The drawing under review shows one solid part. Ordinate dimensions are in mm from its lowest x, y, z. Give positions to 0.01 mm unless a question says otherwise; leave off trailing zeros. Order: outer loops, then holes, each group sorted by start corner. A loop starts at its lowest first (then second) coordinate and runs counter-clockwise, first axis right, second up. Notation, with made-up numbers: (72, 30.5) -> (113, 30.5) arc R23 ccw to (113, 49.5) -> close; hole circle Ø3 at (-5, -9). An arc over 180 degrees is marked (long way). One line per item, written item: value.
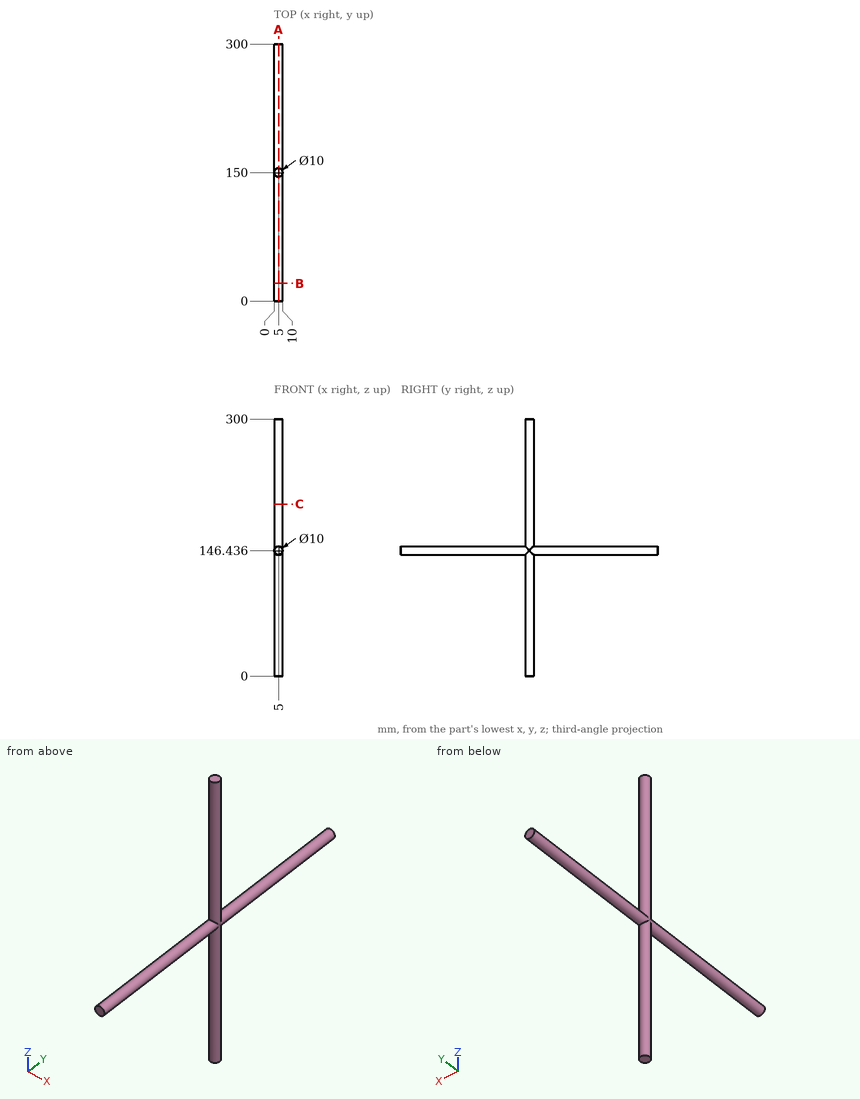
Item 1: Add section C-C on z = 200.5. Give the boundary of the cut face in (x, y).
Returned:
outline: circle Ø10 at (5, 150)
Item 2: Add section A-A on x = 5. Give the boundary of the cut face in (y, z) (1 decimal).
Returned:
outline: (0, 141.4) -> (145, 141.4) -> (145, 0) -> (155, 0) -> (155, 141.4) -> (300, 141.4) -> (300, 151.4) -> (155, 151.4) -> (155, 300) -> (145, 300) -> (145, 151.4) -> (0, 151.4) -> close
Item 3: To check wall thickness, follow line 1 along Z through (x, y) = (5.75, 99.5); line 2 along Y through (x, z) = (5, 135); line 3 along Y through (x, z) = (4.25, 154.5). State the ranges of each line that lie inside material, in increasing order. Write a range as from..to.
Returned:
line 1: 141.49..151.38
line 2: 145..155
line 3: 145.06..154.94
Item 4: Clearance check with flat-ended pins moving along their axes: P1, Ø6, axis at x = 1.5, y = 206, coming from the -Z side; P2, Ø6, axis at x = 4.5, z = 221, coming from the -Y side; P3, Ø4, axis at x = 8.5, z = 41, coming from the -Y side. State where each tip first meets the part, or that it passes through.
Returned:
P1: z = 141.46
P2: y = 145
P3: y = 145.23
Item 5: Add section B-B on y = 20.5. Give the boundary of the cut face in (x, z) (1 decimal).
Returned:
outline: circle Ø10 at (5, 146.4)
